Verification items for this drawing (mm, ordinates from the low corner). Round coordinates to 2 decimals unless told otherwise and drop trailing zeros. Order: outer loops, then holes, each group sorted by start corner. A loop starts at its lowest first (then second) coordinate and runs counter-clockwise, first axis right, second up. Notation, with made-up numbers: M 43,37 L 81,37 A27 cw 81,61 Z; hole C -20,-15 d7. An arc over 180 degrees is marked long. Use CSV: the item, a comma, the result in double quotes. Start each with the question number.
Q1. Sectioned sample at A-A (x = 32.5). Enter the section's corners in (y, z).
Q2. Sectioned sample at B-B (z = 10). Enter the section's corners in (x, y).
Q3. Scan lines: line 1 (X direction, y = 13, z = 10); line 2 (Z direction, x = 32.5, y = 13.25); line 3 (X direction, y = 18.25, z = 10.75). Record each from-to range of solid material in increasing order.
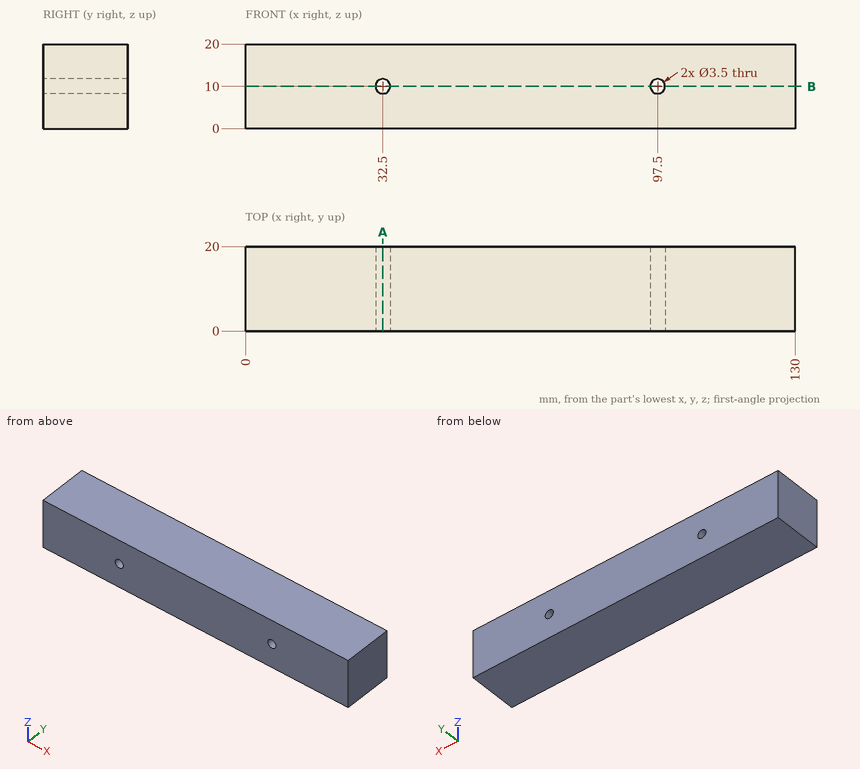
Verdict:
1,outline,"M 0,0 L 20,0 L 20,8.25 L 0,8.25 Z; M 0,11.75 L 20,11.75 L 20,20 L 0,20 Z"
2,outline,"M 0,0 L 30.75,0 L 30.75,20 L 0,20 Z; M 34.25,0 L 95.75,0 L 95.75,20 L 34.25,20 Z; M 99.25,0 L 130,0 L 130,20 L 99.25,20 Z"
3,line 1,"x = 0 to 30.75, 34.25 to 95.75, 99.25 to 130"
3,line 2,"z = 0 to 8.25, 11.75 to 20"
3,line 3,"x = 0 to 30.92, 34.08 to 95.92, 99.08 to 130"
